```python
from build123d import *

# Parameters (mm, degrees)
CUT_EXTRUDE1_DEPTH = 1.3


with BuildPart() as part:
    # Sketch1 → Revolve1 (revolve)
    with BuildSketch(Plane(origin=(0, 0, 0), x_dir=(0, 0, -1), z_dir=(1, 0, 0))):
        with BuildLine():
            Line((0, 0), (0, 2.45))
            Line((0, 2.45), (0.3, 2.75))
            Line((0.3, 2.75), (2.785, 2.75))
            Line((2.785, 2.75), (3, 2.535))
            Line((3, 2.535), (3, 1.8))
            ThreePointArc((3, 1.8), (3.015193643, 1.74701055), (3.056157637, 1.710123155))
            Line((3.056157637, 1.710123155), (3.466157637, 1.510123155))
            ThreePointArc((3.466157637, 1.510123155), (3.48750205, 1.50256365), (3.51, 1.5))
            Line((3.51, 1.5), (27.75, 1.5))
            Line((27.75, 1.5), (28, 1.25))
            Line((28, 1.25), (28, 0))
            Line((28, 0), (0, 0))
        make_face()
    revolve(axis=Axis((0, 0, 0), (0, 0, -1)))

    # Sketch2 → Cut-Extrude1 (cut)
    with BuildSketch(Plane.XY):
        Polygon((0, 1.443375673), (-1.25, 0.721687836), (-1.25, -0.721687836), (0, -1.443375673), (1.25, -0.721687836), (1.25, 0.721687836), align=None)
    extrude(amount=-CUT_EXTRUDE1_DEPTH, mode=Mode.SUBTRACT)

    # Sketch3 → Cut-Revolve2 (revolve, cut)
    with BuildSketch(Plane(origin=(0, 0, 0), x_dir=(0, 0, -1), z_dir=(1, 0, 0))):
        Polygon((1.3, 0), (1.3, 1.25), (2.021687836, 0), align=None)
    revolve(axis=Axis((0, 0, -1.3), (0, 0, -1)), mode=Mode.SUBTRACT)

    # Sketch4 → Cut-Revolve3 (revolve, cut)
    with BuildSketch(Plane(origin=(0, 0, 0), x_dir=(0, 0, -1), z_dir=(1, 0, 0))):
        Polygon((0, 1.443375673), (0, 1.25), (0.051814855, 1.25), align=None)
    revolve(axis=Axis((0, 0, 0), (0, 0, -1)), mode=Mode.SUBTRACT)


solid = part.part
```
Source: CAD feature listing. Evaluate the final solid. Frame: model axes, mm. A direction names the side the tool comes from. Coordinates: 2 decimals unless noted, no trailing zeros. Loops run counter-clockwise (first coordinate to the right, second up) from the corner with the lowest first, then second, coordinate; pieces in that order, holes last. Notation, with made-up numbers: M 6,57.25 L 63,57.25 A11 cw 63,63.25 Z; hole C 58.25,-22.5 d3. An arc over 180 degrees is marked long. Put each result on its own line as item: value. Start each with the question number.
1) Cut plane A-A on z = -21.5. Return the cut outline in (x, y), then the cut area to 3 significant figures.
2) Pull-direction query (X, two-part tool) for faces 1 (the face through (-0.63, -1.08, -0.64)), 2 (the face through (-2, 0, 0)), 3 (the face through (-0.616, 1.088, -0.641)), 4 (the face through (0.07, -1.5, -15.8)); classes: pulls with the +X half, pulls with the -X half, needs draft (parallel to the pull), parting line crosses it, or undercut.
3) Contact query for flat-ended pins moving along their axis: pin 1 Ø1.5 at (x, y) = (-2, 0.5) entering from -Z; pin 2 Ø3 at (y, z) = (-2, -24.5) entering from -X; pin 3 Ø0.7 at (x, y) = (1, 0.5) entering from +Z; pin 4 Ø1 at (x, y) = (-0.5, -0.5) entering from +Z. Output: stop coordinate, or through.
4) Reachability of faces 5 (the face through (-1, -2, -3)), 6 (the face through (0.63, 1.08, -0.64)), 7 (the face through (-2.685, -0.596, -1.56)) from +Z, -Z, +X, -X, +Y, -Y: full face, straight path, thin tool, end or side. Return the list, or none.
5) Ray query, L1, parallel to X at y = -0.4, z = -11.25; L2, parallel to Z at x = 1.7, y = -1.1; L3, parallel to X at y = -0.05, z = -5. Return the intervals inside material, ascending. Write a range as from..to.
The answers:
1. outline: C 0,0 d3
1. area: 7.07 mm²
2. face 1: undercut
2. face 2: needs draft
2. face 3: undercut
2. face 4: parting line crosses it
3. pin 1: stops at z = -27.94
3. pin 2: stops at x = -1.41
3. pin 3: stops at z = 0
3. pin 4: stops at z = -1.32
4. face 5: -Z
4. face 6: +Z
4. face 7: +Z, -Z
5. L1: x = -1.45..1.45
5. L2: z = -3..0
5. L3: x = -1.5..1.5
